from build123d import *

# Parameters (mm, degrees)
F1_DEPTH = 18
F3_DEPTH = 25
F4_R     = 20


with BuildPart() as f1:
    # F0 (on Top) → F1 (new body)
    with BuildSketch(Plane.XY):
        Polygon((158.1674836576, 528.3263906837), (-91.8325163424, 528.3263906837), (-91.8325163424, -71.6736093163), (-56.8325163424, -71.6736093163), (-56.8325163424, -81.6736093163), (-6.8325163424, -81.6736093163), (-6.8325163424, -71.6736093163), (73.1674836576, -71.6736093163), (73.1674836576, -81.6736093163), (123.1674836576, -81.6736093163), (123.1674836576, -71.6736093163), (158.1674836576, -71.6736093163), align=None)
    extrude(amount=F1_DEPTH)

    # F2 (on face) → F3 (cut)
    with BuildSketch(Plane.XY.offset(18)):
        Polygon((158.1674836576, 528.3263906837), (-41.8325163424, 528.3263906837), (-41.8325163424, 453.3263906837), (83.1674836576, 28.3263906837), (158.1674836576, 28.3263906837), align=None)
    extrude(amount=-F3_DEPTH, mode=Mode.SUBTRACT)

    # F4
    f4_edges = [f1.edges().sort_by_distance(p)[0] for p in [
        (-41.832516, 528.326391, 9),
        (158.167484, 28.326391, 9),
        (-41.832516, 453.326391, 9),
        (83.167484, 28.326391, 9),
    ]]
    fillet(f4_edges, radius=F4_R)


solid = f1.part
The listing builds one solid part. Answer for the finished solid, in the listing's coordinates (mm). A direction names the side the tool comes from. Give positions to 0.01 mm unless a question says otherwise; leave off trailing zeros. Loops run counter-clockwise (first coordinate to the right, second up) from the corner with the lowest first, then second, coordinate; pieces in that order, holes last. Notation, with made-up numbers: M -22,47.25 L -10,47.25 A25 ccw -10,86.25 Z; hole C 35.5,67 d6. An arc over 180 degrees is marked long. Answer as CSV lines item,"result".
Item 1: Which of the six approach directions +Z, -Z, +X, -X, +Y, -Y give full straight-line access (tool end or side, diameter ignored) to faces 4 (the flat face through (-56.833, -77, 9)), 5 (the flat face through (33, -71.674, 9)), 6 (the flat face through (118, 28.326, 9)), 7 (the flat face through (140, -71.674, 9))?
Values follow:
face 4,"+Z, -Z, -X, -Y"
face 5,"+Z, -Z, -Y"
face 6,"+Z, -Z, +X, +Y"
face 7,"+Z, -Z, +X, -Y"
Item 2: The mould has two halves that part along X. Classify faces 1 (the flat face through (73.167, -77, 9)), 2 (the flat face through (-32, -81.674, 9)), 3 (the flat face through (-41.833, 483, 9)): released by +X, released by -X, zero draft, split by the parting line, or undercut.
Values follow:
face 1,"undercut"
face 2,"zero draft"
face 3,"released by +X"
Item 3: The part is cut by section B-B (y = 487). Give the vertices of the cut face in (x, z).
Values follow:
outline,"M -91.83,0 L -41.83,0 L -41.83,18 L -91.83,18 Z"
Item 4: Given pin 1 Ø3 at (y, z) = (-74, 12) entering from +X; pin 2 Ø6 at (y, z) = (179, 15) entering from +X; pin 3 Ø5.5 at (y, z) = (492, 11) entering from +X; pin 4 Ø3 at (x, y) = (-14, 76) entering from -Z, each flat-ended and moving along its own axis, determine where each tip first touches the part or whether it passes through.
Values follow:
pin 1,"stops at x = 123.17"
pin 2,"stops at x = 39.73"
pin 3,"stops at x = -41.83"
pin 4,"stops at z = 0"
Item 5: Straight lines are drawn through the part: line 1 along X through (y, z) = (490.5, 17); line 2 along Y through (x, z) = (-60, 5.25); line 3 along Y through (x, z) = (-53, 13.75). For each, find the intervals that lie inside material, in ascending order. Write a range as [from, to].
Values follow:
line 1,"x = [-91.83, -41.83]"
line 2,"y = [-71.67, 528.24]"
line 3,"y = [-81.67, 526.27]"
Item 6: The part is cut by section A-A (z = 11.75). Give the vertices of the cut face in (x, y).
Values follow:
outline,"M -91.83,-71.67 L -56.83,-71.67 L -56.83,-81.67 L -6.83,-81.67 L -6.83,-71.67 L 73.17,-71.67 L 73.17,-81.67 L 123.17,-81.67 L 123.17,-71.67 L 158.17,-71.67 L 158.17,8.33 A20 ccw 138.17,28.33 L 98.13,28.33 A20 cw 78.94,42.68 L -41.02,450.56 A20 cw -41.83,456.21 L -41.83,508.33 A20 ccw -61.83,528.33 L -91.83,528.33 Z"
Item 7: The part is cut by section C-C (x = 63). Give the vertices of the cut face in (y, z).
Values follow:
outline,"M -71.67,0 L 96.9,0 L 96.9,18 L -71.67,18 Z"
